Model file for the job. Use its own axes, mm. Coordinates: 2 decimals unless noted, no trailing zeros. Write each loop counter-clockwise with the first axis right and the second up, starting at its lowest first coordinate (ties: lowest second). Pieces come first, ordered by that corner, then holes. Notation, with made-up numbers: (63.25, 69.5) - (113.25, 69.5) arc R13 cw to (113.25, 81.5) - close; hole circle Ø2 at (-29.75, 42.5). An arc over 180 degrees is marked (long way). Put each result on its own line as item: value. Start each with the question number.
1. Drop flat-ended pins along their axis: P1, Ø6, axis at x = 11.5, z = -19.5, coming from the -Y side; P2, Ø3, axis at y = 15, z = -54, coming from the +X side; P3, Ø3, axis at x = -2.5, z = -51, coming from the +Y side. Give the stop position or say it passes through.
2. Saw through at B-B, the plane x = -3. Write the cut outline in (y, z).
3. Saw through at A-A, the plane z = -65.85. Write the cut outline in (x, y).
4. Saw through at C-C, the plane z = -19. Write the cut outline in (x, y), plus the area to 3 significant figures.
5. Saw through at D-D, the plane y = 16.75. Write the cut outline in (x, z), plus the area to 3 significant figures.
6. Drill centre lines: L1, parallel to X at y = 10.75, z = -65.85; L2, parallel to X at y = 25.75, z = -80.5; L3, parallel to Y at x = 9.25, z = -74.5. Where is each one in solid material? Low to high. Write a range as from..to.
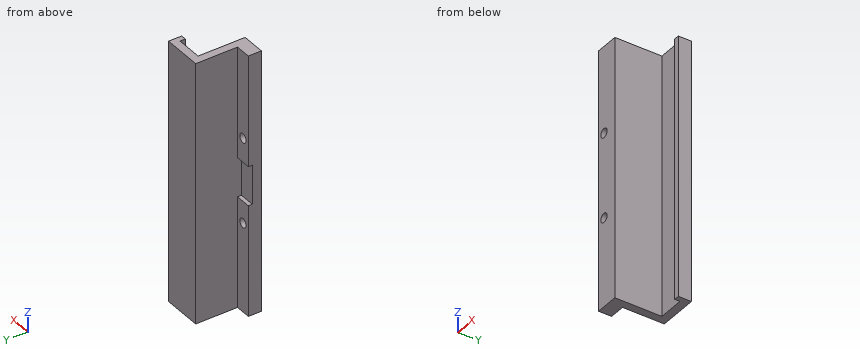
```python
from build123d import *

# Parameters (mm, degrees)
SKETCH1_W            = 100
SKETCH1_H            = 26
BOSS_EXTRUDE1_DEPTH  = 2
BOSS_EXTRUDE2_DEPTH  = 100
MOVE_START           = -100
MOVE_FACE1_OUTLINE_W = 2
MOVE_FACE1_OUTLINE_H = 28
MOVE_FACE1_DEPTH     = 100
SKETCH5_W            = 100
SKETCH5_H            = 4
BOSS_EXTRUDE3_DEPTH  = 6
SKETCH6_W            = 100
SKETCH6_H            = 4
BOSS_EXTRUDE4_DEPTH  = 4
SKETCH7_W            = 6
SKETCH7_H            = 100
BOSS_EXTRUDE5_DEPTH  = 11.5
MOVE_FACE2_BY        = 12
SKETCH8_W            = 6
SKETCH8_H            = 42.5
BOSS_EXTRUDE6_DEPTH  = 1.5
SKETCH9_R            = 1.75
CUT_EXTRUDE1_DEPTH   = 103.376755174
MOVE_FACE3_BY        = 1
MOVE_FACE3_2_BY      = 1
MOVE_FACE3_3_BY      = 1
MOVE_FACE4_BY        = 1


# Read off the part's stored shape, not the designer's step: Move Face1
with BuildPart() as part:
    # Sketch1 → Boss-Extrude1 (new body)
    with BuildSketch(Plane(origin=(0, 0, 0), x_dir=(0, 0, -1), z_dir=(1, 0, 0))):
        with Locations((50, 13)):
            Rectangle(SKETCH1_W, SKETCH1_H)
    extrude(amount=BOSS_EXTRUDE1_DEPTH)

    # Sketch2 → Boss-Extrude2 (add)
    with BuildSketch(Plane.XY):
        Polygon((2, 26), (2, 28), (-12, 28), (-12, 24), (-10, 24), (-10, 26), align=None)
    extrude(amount=-BOSS_EXTRUDE2_DEPTH)


with BuildPart() as body_2:
    # Mirror1: mirrored copy
    add(part.part.mirror(Plane.ZY.offset(-2)))

    # Move Face1 outline → Move Face1 (add)
    with BuildSketch(Plane.XY.offset(MOVE_START)):
        with Locations((1, 14)):
            Rectangle(MOVE_FACE1_OUTLINE_W, MOVE_FACE1_OUTLINE_H)
    extrude(amount=MOVE_FACE1_DEPTH)



with BuildPart() as body_2_2:
    # Sketch5 → Boss-Extrude3 (new body)
    with BuildSketch(Plane.ZY):
        with Locations((-50, -2)):
            Rectangle(SKETCH5_W, SKETCH5_H)
    extrude(amount=BOSS_EXTRUDE3_DEPTH)


with BuildPart() as body_2_1:
    add(body_2.part)

    add(body_2_2.part)  # Boss-Extrude4 merges body 2 2
    # Sketch6 → Boss-Extrude4 (add)
    with BuildSketch(Plane(origin=(0, 0, 0), x_dir=(0, 0, -1), z_dir=(1, 0, 0))):
        with Locations((50, -2)):
            Rectangle(SKETCH6_W, SKETCH6_H)
    extrude(amount=BOSS_EXTRUDE4_DEPTH)

    # Sketch7 → Boss-Extrude5 (add)
    with BuildSketch(Plane(origin=(0, 0, 0), x_dir=(1, 0, 0), z_dir=(0, 1, 0))):
        with Locations((-3, 50)):
            Rectangle(SKETCH7_W, SKETCH7_H)
    extrude(amount=BOSS_EXTRUDE5_DEPTH)

    # Move Face2: a face moved inward by 12.0
    extrude(body_2_1.faces().sort_by_distance((-1, -4, -50))[0], amount=MOVE_FACE2_BY, dir=(0, 1, 0), mode=Mode.SUBTRACT)

    # Sketch8 → Boss-Extrude6 (add)
    with BuildSketch(Plane(origin=(0, 11.5, 0), x_dir=(1, 0, 0), z_dir=(0, 1, 0))):
        with Locations((-3, 78.75)):
            Rectangle(SKETCH8_W, SKETCH8_H)
        with Locations((-3, 21.25)):
            Rectangle(SKETCH8_W, SKETCH8_H)
    extrude(amount=BOSS_EXTRUDE6_DEPTH)

    # Sketch9 → Cut-Extrude1 (cut, through all)
    with BuildSketch(Plane(origin=(0, 13, 0), x_dir=(1, 0, 0), z_dir=(0, 1, 0))):
        with Locations(Location((-3, 33.28320942, 0), (0, 0, 270))):
            Circle(SKETCH9_R)
        with Locations(Location((-3, 65.85, 0), (0, 0, 270))):
            Circle(SKETCH9_R)
    extrude(amount=-CUT_EXTRUDE1_DEPTH, mode=Mode.SUBTRACT)

    # Move Face3: a face moved inward by 1.0
    extrude(body_2_1.faces().sort_by_distance((16, 26, -50))[0], amount=MOVE_FACE3_BY, dir=(-1, 0, 0), mode=Mode.SUBTRACT)

    # Move Face3 2: a face moved inward by 1.0
    extrude(body_2_1.faces().sort_by_distance((4, 17, -50))[0], amount=MOVE_FACE3_2_BY, dir=(-1, 0, 0), mode=Mode.SUBTRACT)

    # Move Face3 3: a face moved outward by 1.0
    extrude(body_2_1.faces().sort_by_distance((14, 25, -50))[0], amount=MOVE_FACE3_3_BY, dir=(-1, 0, 0))

    # Move Face4: a face moved outward by 1.0
    extrude(body_2_1.faces().sort_by_distance((7.5, 28, -50))[0], amount=MOVE_FACE4_BY, dir=(0, 1, 0))


solid = body_2_1.part
```
Final values:
1. P1: stops at y = 24
1. P2: stops at x = 3
1. P3: stops at y = 11.5
2. outline: (8, -100) - (13, -100) - (13, -67.6) - (8, -67.6) - close; (8, -64.1) - (13, -64.1) - (13, -57.5) - (11.5, -57.5) - (11.5, -42.5) - (13, -42.5) - (13, -35.03) - (8, -35.03) - close; (8, -31.53) - (13, -31.53) - (13, 0) - (8, 0) - close
3. outline: (-6, 8) - (-4.75, 8) - (-4.75, 13) - (-6, 13) - close; (-1.25, 8) - (3, 8) - (3, 26) - (13, 26) - (13, 24) - (15, 24) - (15, 29) - (0, 29) - (0, 13) - (-1.25, 13) - close
4. outline: (-6, 8) - (3, 8) - (3, 26) - (13, 26) - (13, 24) - (15, 24) - (15, 29) - (0, 29) - (0, 13) - (-6, 13) - close
4. area: 133 mm²
5. outline: (0, -100) - (3, -100) - (3, 0) - (0, 0) - close
5. area: 300 mm²
6. L1: x = -6..-4.75, -1.25..3
6. L2: x = 0..3, 13..15
6. L3: y = 26..29
